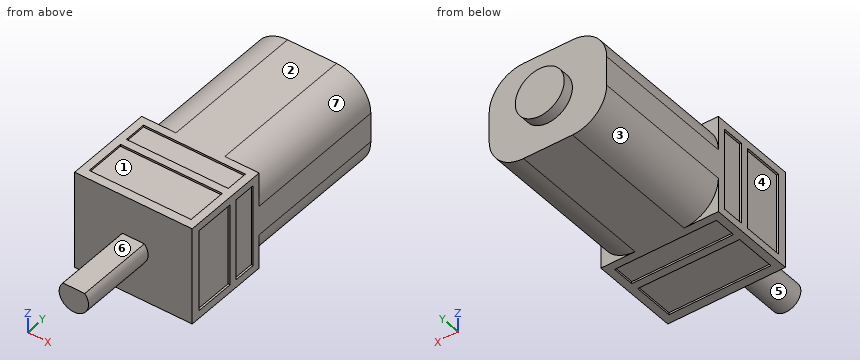
from build123d import *

# Parameters (mm, degrees)
SKETCH1_W           = 12
SKETCH1_H           = 10
BOSS_EXTRUDE1_DEPTH = 9
BOSS_EXTRUDE2_DEPTH = 15
SKETCH3_R           = 2.5
BOSS_EXTRUDE3_DEPTH = 1.1
BOSS_EXTRUDE4_DEPTH = 8
SKETCH5_W           = 10.4
SKETCH5_H           = 2.3
SKETCH5_H_2         = 4.2
CUT_EXTRUDE1_DEPTH  = 0.2
SKETCH6_W           = 8.4
SKETCH6_H           = 2.3
SKETCH6_H_2         = 4.2
CUT_EXTRUDE2_DEPTH  = 0.2


with BuildPart() as part:
    # Sketch1 → Boss-Extrude1 (new body)
    with BuildSketch(Plane(origin=(0, 0, 0), x_dir=(1, 0, 0), z_dir=(0, 1, 0))):
        Rectangle(SKETCH1_W, SKETCH1_H)
    extrude(amount=BOSS_EXTRUDE1_DEPTH)

    # Sketch2 → Boss-Extrude2 (add)
    with BuildSketch(Plane(origin=(0, 9, 0), x_dir=(1, 0, 0), z_dir=(0, 1, 0))):
        with BuildLine():
            Line((-2.5, 5), (2.5, 5))
            ThreePointArc((2.5, 5), (4.974873734, 3.974873734), (6, 1.5))
            Line((6, 1.5), (6, -1.5))
            ThreePointArc((6, -1.5), (4.974873734, -3.974873734), (2.5, -5))
            Line((2.5, -5), (-2.5, -5))
            ThreePointArc((-2.5, -5), (-4.974873734, -3.974873734), (-6, -1.5))
            Line((-6, -1.5), (-6, 1.5))
            ThreePointArc((-6, 1.5), (-4.974873734, 3.974873734), (-2.5, 5))
        make_face()
    extrude(amount=BOSS_EXTRUDE2_DEPTH)

    # Sketch3 → Boss-Extrude3 (add)
    with BuildSketch(Plane(origin=(0, 24, 0), x_dir=(1, 0, 0), z_dir=(0, 1, 0))):
        Circle(SKETCH3_R)
    extrude(amount=BOSS_EXTRUDE3_DEPTH)

    # Sketch4 → Boss-Extrude4 (add)
    with BuildSketch(Plane.XZ):
        with BuildLine():
            Line((-1.118033989, 1), (1.118033989, 1))
            ThreePointArc((1.118033989, 1), (0, -1.5), (-1.118033989, 1))
        make_face()
    extrude(amount=BOSS_EXTRUDE4_DEPTH)

    # Sketch5 → Cut-Extrude1 (cut)
    with BuildSketch(Plane.XY.offset(5)):
        with Locations((0, 7.05)):
            Rectangle(SKETCH5_W, SKETCH5_H)
        with Locations((0, 3)):
            Rectangle(SKETCH5_W, SKETCH5_H_2)
    cut_extrude1 = extrude(amount=-CUT_EXTRUDE1_DEPTH, mode=Mode.SUBTRACT)

    # Mirror1: Cut-Extrude1 across plane
    add(cut_extrude1.mirror(Plane.XY), mode=Mode.SUBTRACT)

    # Sketch6 → Cut-Extrude2 (cut)
    with BuildSketch(Plane.ZY.offset(6)):
        with Locations((0, 7.05)):
            Rectangle(SKETCH6_W, SKETCH6_H)
        with Locations((0, 3)):
            Rectangle(SKETCH6_W, SKETCH6_H_2)
    cut_extrude2 = extrude(amount=-CUT_EXTRUDE2_DEPTH, mode=Mode.SUBTRACT)

    # Mirror2: Cut-Extrude2 across plane
    add(cut_extrude2.mirror(Plane(origin=(0, 0, 0), x_dir=(0, 0, 1), z_dir=(1, 0, 0))), mode=Mode.SUBTRACT)


solid = part.part
Geometry check sheet. Reference: the model listing, model coordinates, mm. Face numbers are marked on the shaded views. A direction names the side the tool comes from. Give positions to 0.01 mm unless a question says otherwise; leave off trailing zeros. Loops run counter-clockwise (first coordinate to the right, second up) from the corner with the lowest first, then second, coordinate; pieces in that order, holes last.
(1) Release check for a two-part mould opening along X. For the marked faces 1, 2 and 3 record: released by +X, released by -X, zero draft, split by the parting line, or undercut.
From the geometry:
face 1: undercut
face 2: zero draft
face 3: released by -X
(2) Section check D-D on z = 3. Record the cut outline in (x, y), then the cut area to 3 significant figures.
From the geometry:
outline: (-6, 0) - (6, 0) - (6, 0.9) - (5.8, 0.9) - (5.8, 5.1) - (6, 5.1) - (6, 5.9) - (5.8, 5.9) - (5.8, 8.2) - (6, 8.2) - (6, 9) - (5.66, 9) - (5.66, 24) - (-5.66, 24) - (-5.66, 9) - (-6, 9) - (-6, 8.2) - (-5.8, 8.2) - (-5.8, 5.9) - (-6, 5.9) - (-6, 5.1) - (-5.8, 5.1) - (-5.8, 0.9) - (-6, 0.9) - close
area: 275 mm2
(3) Set-up check for the marked faces 4, 5, 6 and 7: record each of +Z, -Z, +X, -X, +Y, -Y from which the full face is reachable in a straight line by a thin tool's end or side.
From the geometry:
face 4: -X
face 5: -Y
face 6: +Z, +X, -X, -Y
face 7: +Z, +X, +Y
(4) Section check B-B on z = 0. Record the cut outline in (x, y), then the cut area to 3 significant figures.
From the geometry:
outline: (-6, 0) - (-1.5, 0) - (-1.5, -8) - (1.5, -8) - (1.5, 0) - (6, 0) - (6, 0.9) - (5.8, 0.9) - (5.8, 5.1) - (6, 5.1) - (6, 5.9) - (5.8, 5.9) - (5.8, 8.2) - (6, 8.2) - (6, 24) - (2.5, 24) - (2.5, 25.1) - (-2.5, 25.1) - (-2.5, 24) - (-6, 24) - (-6, 8.2) - (-5.8, 8.2) - (-5.8, 5.9) - (-6, 5.9) - (-6, 5.1) - (-5.8, 5.1) - (-5.8, 0.9) - (-6, 0.9) - close
area: 315 mm2
(5) Section check A-A on y = 17. Record the cut outline in (x, z), then the cut area to 3 significant figures.
From the geometry:
outline: (-6, -1.5) arc R3.5 ccw to (-2.5, -5) - (2.5, -5) arc R3.5 ccw to (6, -1.5) - (6, 1.5) arc R3.5 ccw to (2.5, 5) - (-2.5, 5) arc R3.5 ccw to (-6, 1.5) - close
area: 109 mm2
(6) Section check C-C on x = 0. Record the cut outline in (y, z).
From the geometry:
outline: (-8, -1.5) - (0, -1.5) - (0, -5) - (0.9, -5) - (0.9, -4.8) - (5.1, -4.8) - (5.1, -5) - (5.9, -5) - (5.9, -4.8) - (8.2, -4.8) - (8.2, -5) - (24, -5) - (24, -2.5) - (25.1, -2.5) - (25.1, 2.5) - (24, 2.5) - (24, 5) - (8.2, 5) - (8.2, 4.8) - (5.9, 4.8) - (5.9, 5) - (5.1, 5) - (5.1, 4.8) - (0.9, 4.8) - (0.9, 5) - (0, 5) - (0, 1) - (-8, 1) - close
(7) Depth check by flat-ended pin: pin 1 Ø1 at (y, z) = (6, -0.5) entering from +X; pin 2 Ø1.8 at (x, z) = (4.5, -3.5) entering from +Y. Enter the tip coordinate at first touch or a pass-through.
From the geometry:
pin 1: stops at x = 6
pin 2: stops at y = 24
(8) Thickness scan on L1, parallel to Y at x = 3, z = 3; L2, parallel to Z at x = 3, y = 6; L3, parallel to Y at x = -2.25, z = 0.25. Record the ranges inside material, lowest first.
From the geometry:
L1: y = 0 to 24
L2: z = -4.8 to 4.8
L3: y = 0 to 25.1
